from build123d import *

# Parameters (mm, degrees)
SKETCH1_R           = 4
BOSS_EXTRUDE1_DEPTH = 55.94
SKETCH2_R           = 6
BOSS_EXTRUDE2_DEPTH = 3
SKETCH3_R           = 0.2
CUT_EXTRUDE1_DEPTH  = 3
CIRPATTERN1_COUNT   = 24


with BuildPart() as part:
    # Sketch1 → Boss-Extrude1 (new body)
    with BuildSketch(Plane(origin=(0, 0, 0), x_dir=(0, 0, -1), z_dir=(1, 0, 0))):
        Circle(SKETCH1_R)
    extrude(amount=BOSS_EXTRUDE1_DEPTH)

    # Sketch2 → Boss-Extrude2 (add)
    with BuildSketch(Plane(origin=(55.94, 0, 0), x_dir=(0, 0, -1), z_dir=(1, 0, 0))):
        Circle(SKETCH2_R)
    extrude(amount=BOSS_EXTRUDE2_DEPTH)

    # Sketch3 → Cut-Extrude1 (cut)
    with BuildSketch(Plane(origin=(58.94, 0, 0), x_dir=(0, 0, -1), z_dir=(1, 0, 0))):
        with Locations((-6, 0)):
            Circle(SKETCH3_R)
    cut_extrude1 = extrude(amount=-CUT_EXTRUDE1_DEPTH, mode=Mode.SUBTRACT)

    # CirPattern1: Cut-Extrude1 ×24 about axis
    cirpattern1_axis = Axis((0, 0, 0), (1, 0, 0))
    for i in range(1, CIRPATTERN1_COUNT):
        add(cut_extrude1.rotate(cirpattern1_axis, i * 360 / CIRPATTERN1_COUNT), mode=Mode.SUBTRACT)


solid = part.part
Verification items for the finished model (mm, model axes). A direction names the side the tool comes from. Give positions to 0.01 mm unless a question says otherwise; leave off trailing zeros. Write each loop counter-clockwise with the first axis right and the second up, starting at its lowest first coordinate (ties: lowest second). Pieces come first, ordered by that corner, then holes. Notation, with made-up numbers: M -37,28 L 10,28 A20 ccw 10,60 Z; hole C -38.5,59 d10. An arc over 180 degrees is marked long. Write item = value, one per line.
(1) Go/stop test with flat-tipped pins: pin 1 Ø5 at (x, z) = (29, 0.5) entering from +Y; pin 2 Ø3 at (x, z) = (35, 2.5) entering from -Y; pin 3 Ø2 at (x, y) = (45, -0.5) entering from +Z. Record where each tip stops, or that it passes through.
Found:
pin_1 = 4
pin_2 = -3.87
pin_3 = 4
(2) Sectioned sample at A-A (x = 45.5). Record the cut outline in (y, z), then the cut area to 3 significant figures.
Found:
outline = C 0,0 d8
area = 50.3 mm2
(3) Material ranges on line 1 (X direction, y = 5, z = -1.75); line 2 (Z direction, x = 50, y = -3.25); line 3 (Y direction, x = 9.5, z = 1), recorded low to high.
Found:
line_1 = 55.94 to 58.94
line_2 = -2.33 to 2.33
line_3 = -3.87 to 3.87
(4) Access from +Z, -Z, +X, -X, +Y, -Y to the whole of each face (thin tool, end or side, straight path). Record for faces 1 (the face through (55.94, 1.42, -3.91)), 2 (the face through (57.419, 0.791, 5.948)).
Found:
face_1 = -X
face_2 = +Z, +X, -X, +Y
